Work out the finished part from the listing and answer in its coordinate system (mm). A direction names the side the tool comes from. Coordinates: 2 decimals unless noted, no trailing zeros. Order: outer loops, then holes, each group sorted by start corner. A loop starts at its lowest first (then second) coordinate and runs counter-clockwise, first axis right, second up. Notation, with made-up numbers: (14, 27.5) -> (50, 27.5) arc R12 cw to (50, 45.5) -> close; hole circle Ø4 at (41, 78.5). An arc over 180 degrees is marked (long way). Use one line per item in the form item = value.
from build123d import *

# Parameters (mm, degrees)
F0_W     = 36.3689862838
F0_H     = 36.3689862838
F1_DEPTH = 2
F2_R     = 2
F3_W     = 20
F3_H     = 20
F4_DEPTH = 25
F5_W     = 2
F5_H     = 21.2931740639
F7_W     = 1.6942393252
F7_H     = 21.2931740639


with BuildPart() as f1:
    # F0 (on Top) → F1 (new body)
    with BuildSketch(Plane.XY):
        Rectangle(F0_W, F0_H)
        with BuildLine():
            ThreePointArc((-15.25, 13.5), (-16.4874368671, 16.4874368671), (-13.5, 15.25))
            Line((-13.5, 15.25), (13.5, 15.25))
            ThreePointArc((13.5, 15.25), (15.25, 17), (17, 15.25))
            ThreePointArc((17, 15.25), (16.4874368671, 14.0125631329), (15.25, 13.5))
            Line((15.25, 13.5), (15.25, -13.5))
            ThreePointArc((15.25, -13.5), (16.4874368671, -14.0125631329), (17, -15.25))
            ThreePointArc((17, -15.25), (15.25, -17), (13.5, -15.25))
            Line((13.5, -15.25), (-13.5, -15.25))
            ThreePointArc((-13.5, -15.25), (-16.4874368671, -16.4874368671), (-15.25, -13.5))
            Line((-15.25, -13.5), (-15.25, 13.5))
        make_face(mode=Mode.SUBTRACT)
        with BuildLine():
            Line((13.5, 15.25), (-13.5, 15.25))
            ThreePointArc((-13.5, 15.25), (-14.0125631329, 14.0125631329), (-15.25, 13.5))
            Line((-15.25, 13.5), (-15.25, -13.5))
            ThreePointArc((-15.25, -13.5), (-14.0125631329, -14.0125631329), (-13.5, -15.25))
            Line((-13.5, -15.25), (13.5, -15.25))
            ThreePointArc((13.5, -15.25), (14.0125631329, -14.0125631329), (15.25, -13.5))
            Line((15.25, -13.5), (15.25, 13.5))
            ThreePointArc((15.25, 13.5), (14.0125631329, 14.0125631329), (13.5, 15.25))
        make_face()
    extrude(amount=F1_DEPTH)

    # F2
    f2_edges = [f1.edges().sort_by_distance(p)[0] for p in [
        (-18.184493, 18.184493, 1),
        (-18.184493, -18.184493, 1),
        (18.184493, 18.184493, 1),
        (18.184493, -18.184493, 1),
    ]]
    fillet(f2_edges, radius=F2_R)

    # F3 (on face) → F4 (cut)
    with BuildSketch(Plane.XY.offset(2)):
        Rectangle(F3_W, F3_H)
    extrude(amount=-F4_DEPTH, mode=Mode.SUBTRACT)

    # F5 (on face) → F8 section 0
    with BuildSketch(Plane.XY.offset(2)):
        with Locations((-12.5, 0)):
            Rectangle(F5_W, F5_H)
    # F7 (on offset) → F8 section 1
    with BuildSketch(Plane.XY.offset(5)):
        with Locations((-9.3471196626, 0)):
            Rectangle(F7_W, F7_H)
    loft()

    # F5 (on face) → F9 section 0
    with BuildSketch(Plane.XY.offset(2)):
        with Locations((12.5, 0)):
            Rectangle(F5_W, F5_H)
    # F7 (on offset) → F9 section 1
    with BuildSketch(Plane.XY.offset(5)):
        with Locations((9.3471196626, 0)):
            Rectangle(F7_W, F7_H)
    loft()


solid = f1.part
(1) Which of the six approach directions +Z, -Z, +X, -X, +Y, -Y give full straight-line access (tool end or side, diameter ignored) to faces 1 (the flat face through (-11.824, 0.149, 3.521)), 2 (the flat face through (0, -10, 1)), 3 (the flat face through (10, 0.1, 3.5))?
Data:
face_1 = +Z, -X, +Y, -Y
face_2 = -Z
face_3 = +Y, -Y
(2) Section B-B on z = 1.05 is taken. Write down the section's boundary in (x, y), plus the area to 3 significant figures.
Data:
outline = (-18.18, -16.18) arc R2 ccw to (-16.18, -18.18) -> (16.18, -18.18) arc R2 ccw to (18.18, -16.18) -> (18.18, 16.18) arc R2 ccw to (16.18, 18.18) -> (-16.18, 18.18) arc R2 ccw to (-18.18, 16.18) -> close; hole circle Ø3.5 at (-15.25, -15.25); hole circle Ø3.5 at (-15.25, 15.25); hole (-10, -10) -> (10, -10) -> (10, 10) -> (-10, 10) -> close; hole circle Ø3.5 at (15.25, -15.25); hole circle Ø3.5 at (15.25, 15.25)
area = 881 mm²
(3) Straight lines are drawn through the part: line 1 along X through (y, z) = (-15.25, 1.1); line 2 along X through (y, z) = (-6, 1.9). For each, find the intervals that lie inside material, in ascending order.
Data:
line_1 = -18.18 to -17, -13.5 to 13.5, 17 to 18.18
line_2 = -18.18 to -10, 10 to 18.18
(4) Section C-C on x = -6 is taken. Write down the section's boundary in (y, z).
Data:
outline = (-18.18, 0) -> (-10, 0) -> (-10, 2) -> (-18.18, 2) -> close; (10, 0) -> (18.18, 0) -> (18.18, 2) -> (10, 2) -> close
(5) The mould has two halves that part along Z. Classify faces 4 (the flat face through (-10, -0.1, 3.5)), 5 (the flat face through (11.824, -0.149, 3.521)), 6 (the flat face through (-10, 0, 1)): released by +Z, released by -Z, zero draft, split by the parting line, or undercut.
Data:
face_4 = undercut
face_5 = released by +Z
face_6 = zero draft
(6) Section A-A on y = 1 is taken. Write down the section's boundary in (x, z).
Data:
outline = (-18.18, 0) -> (-10, 0) -> (-10, 2) -> (-11.5, 2) -> (-8.5, 5) -> (-10.19, 5) -> (-13.5, 2) -> (-18.18, 2) -> close; (8.5, 5) -> (11.5, 2) -> (10, 2) -> (10, 0) -> (18.18, 0) -> (18.18, 2) -> (13.5, 2) -> (10.19, 5) -> close
(7) This flat-tipped pin is pushed along its axis until it touches: P1, Ø5, axis at x = -5.5, y = 1, coming from the -Z side. Where does it stop, or does it pass through?
Data:
P1 = through
